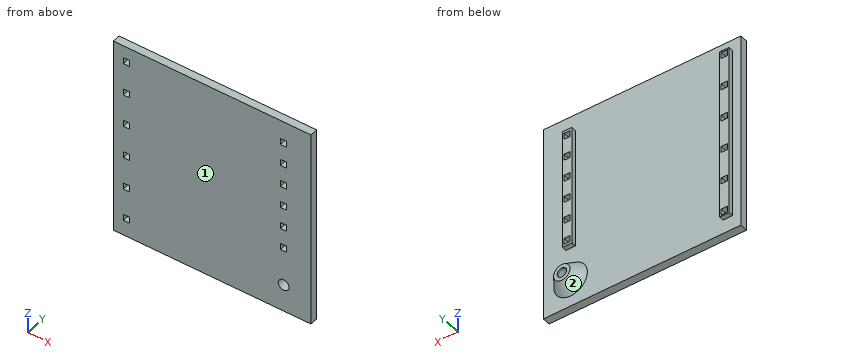
from build123d import *

# Parameters (mm, degrees)
SKETCH1_W           = 126
SKETCH1_H           = 126
BOSS_EXTRUDE1_DEPTH = 5
SKETCH3_R           = 12.5
BOSS_EXTRUDE2_DEPTH = 7.5
SKETCH4_R           = 3.45
CUT_EXTRUDE1_DEPTH  = 11.5
SKETCH6_R           = 3
CUT_EXTRUDE2_DEPTH  = 179.628805068
CHAMFER1_SIZE       = 10
CHAMFER1_SIZE_2     = 7.26542528
SKETCH9_W           = 6
SKETCH9_H           = 77
BOSS_EXTRUDE4_DEPTH = 3
SKETCH10_W          = 4
SKETCH10_H          = 4
CUT_EXTRUDE4_DEPTH  = 179.370401132
SKETCH11_W          = 6
SKETCH11_H          = 110
BOSS_EXTRUDE5_DEPTH = 3
SKETCH12_W          = 4
SKETCH12_H          = 4
CUT_EXTRUDE5_DEPTH  = 179.370401132


with BuildPart() as part:
    # Sketch1 → Boss-Extrude1 (new body)
    with BuildSketch(Plane(origin=(0, 0, 0), x_dir=(1, 0, 0), z_dir=(0, 1, 0))):
        with Locations((63, 63)):
            Rectangle(SKETCH1_W, SKETCH1_H)
    extrude(amount=BOSS_EXTRUDE1_DEPTH)

    # Sketch3 → Boss-Extrude2 (add)
    with BuildSketch(Plane(origin=(0, 5, 0), x_dir=(1, 0, 0), z_dir=(0, 1, 0))):
        with Locations(Location((108.6, 108.6, 0), (0, 0, 90))):
            Circle(SKETCH3_R)
    extrude(amount=BOSS_EXTRUDE2_DEPTH)

    # Sketch4 → Cut-Extrude1 (cut)
    with BuildSketch(Plane.XZ):
        with Locations(Location((108.6, -108.6, 0), (0, 0, 270))):
            Circle(SKETCH4_R)
    extrude(amount=-CUT_EXTRUDE1_DEPTH, mode=Mode.SUBTRACT)

    # Sketch6 → Cut-Extrude2 (cut, through all)
    with BuildSketch(Plane(origin=(0, 12.5, 0), x_dir=(1, 0, 0), z_dir=(0, 1, 0))):
        with Locations(Location((108.6, 108.6, 0), (0, 0, 270))):
            Circle(SKETCH6_R)
    extrude(amount=-CUT_EXTRUDE2_DEPTH, mode=Mode.SUBTRACT)

    # Chamfer1
    # the kernel refuses this chamfer: 10, 7.26542528 mm, written as the material it takes off along each edge
    with BuildSketch(Plane(origin=(108.6, 12.5, -108.6), x_dir=(0, 0, -1), z_dir=(1, 0, 0))) as chamfer1_piece_1_section:
        Polygon((12.5, -CHAMFER1_SIZE), (12.5 - CHAMFER1_SIZE_2, 0), (12.5, 0), align=None)
    chamfer1_piece_1 = revolve(axis=Axis((108.6, 12.5, -108.6), (0, 1, 0)), mode=Mode.PRIVATE)
    chamfer1_piece_1 = split(chamfer1_piece_1, bisect_by=Plane(origin=(108.6, 5, -100.650989912), z_dir=(0, 1, 0)), keep=Keep.TOP, mode=Mode.PRIVATE)
    add(chamfer1_piece_1, mode=Mode.SUBTRACT)

    # Sketch9 → Boss-Extrude4 (add)
    with BuildSketch(Plane(origin=(0, 5, 0), x_dir=(1, 0, 0), z_dir=(0, 1, 0))):
        with Locations((108.6, 48.95817816)):
            Rectangle(SKETCH9_W, SKETCH9_H)
    extrude(amount=BOSS_EXTRUDE4_DEPTH)

    # Sketch10 → Cut-Extrude4 (cut, through all)
    with BuildSketch(Plane(origin=(0, 8, 0), x_dir=(1, 0, 0), z_dir=(0, 1, 0))):
        with Locations((108.6, 83.95817816)):
            Rectangle(SKETCH10_W, SKETCH10_H)
        with Locations((108.6, 69.958932274)):
            Rectangle(SKETCH10_W, SKETCH10_H)
        with Locations((108.6, 55.959686388)):
            Rectangle(SKETCH10_W, SKETCH10_H)
        with Locations((108.6, 41.960440502)):
            Rectangle(SKETCH10_W, SKETCH10_H)
        with Locations((108.6, 27.961194616)):
            Rectangle(SKETCH10_W, SKETCH10_H)
        with Locations((108.6, 13.96194873)):
            Rectangle(SKETCH10_W, SKETCH10_H)
    extrude(amount=-CUT_EXTRUDE4_DEPTH, mode=Mode.SUBTRACT)

    # Sketch11 → Boss-Extrude5 (add)
    with BuildSketch(Plane(origin=(0, 5, 0), x_dir=(1, 0, 0), z_dir=(0, 1, 0))):
        with Locations((8.381061813, 62)):
            Rectangle(SKETCH11_W, SKETCH11_H)
    extrude(amount=BOSS_EXTRUDE5_DEPTH)

    # Sketch12 → Cut-Extrude5 (cut, through all)
    with BuildSketch(Plane(origin=(0, 8, 0), x_dir=(1, 0, 0), z_dir=(0, 1, 0))):
        with Locations((8.381061813, 114.236582212)):
            Rectangle(SKETCH12_W, SKETCH12_H)
        with Locations((8.381061813, 93.358892092)):
            Rectangle(SKETCH12_W, SKETCH12_H)
        with Locations((8.381061813, 72.481201972)):
            Rectangle(SKETCH12_W, SKETCH12_H)
        with Locations((8.381061813, 51.603511852)):
            Rectangle(SKETCH12_W, SKETCH12_H)
        with Locations((8.381061813, 30.725821731)):
            Rectangle(SKETCH12_W, SKETCH12_H)
        with Locations((8.381061813, 9.848131611)):
            Rectangle(SKETCH12_W, SKETCH12_H)
    extrude(amount=-CUT_EXTRUDE5_DEPTH, mode=Mode.SUBTRACT)


solid = part.part
Work out the finished part from the listing and answer in its coordinate system (mm). Face numbers are marked on the shaded views. Coordinates: 2 decimals unless noted, no trailing zeros. Loops run counter-clockwise (first coordinate to the right, second up) from the corner with the lowest first, then second, coordinate; pieces in that order, holes last. Notation, with made-up numbers: M 52,5.5 L 90,5.5 A17 ccw 90,32.5 Z; hole C 20.5,-3.5 d5. An arc over 180 degrees is marked long. Answer in a Markdown table with one row per item. Add a question column.
1. Find section C-C, the plane z = -78.5. Write down the section's boundary in (x, y).
2. Find section D-D, the plane x = 66. Write down the section's boundary in (y, z).
3. Find section A-A, the plane z = -108.6. Write down the section's boundary in (x, y).
4. Consider L1, parallel to X at y = 4, z = -108.6; L2, parallel to X at y = 6.5, z = -34; L3, parallel to Y at x = 99.5, z = -93. Determine where each line is inside the solid, lowest interval first.
5. Flat-ended cylindrical pins translate along their axes: P1, Ø1.5, axis at y = 10, z = -111.5, coming from the -X side; P2, Ø2.5, axis at x = 109.5, y = 6.5, coming from the -Z side; P3, Ø2, axis at x = 37.5, z = -71.5, coming from the +Y side. Find the tip coordinate at first contact, or state that the pin passes through.
6. The mould has two halves that part along X. Classify the marked faces 1 and 2: pulls with the +X half, pulls with the -X half, needs draft (parallel to the pull), parting line crosses it, or undercut.
7. Find section B-B, the plane x = 108.6. State how many separate pieces and enclosed holes the cut face has, then the cut area to 3 significant figures.
Reported:
| question | item | result |
|---|---|---|
| 1 | outline | M 0,0 L 126,0 L 126,5 L 111.6,5 L 111.6,8 L 105.6,8 L 105.6,5 L 11.38,5 L 11.38,8 L 5.38,8 L 5.38,5 L 0,5 Z |
| 2 | outline | M 0,-126 L 5,-126 L 5,0 L 0,0 Z |
| 3 | outline | M 0,0 L 105.15,0 L 105.15,11.5 L 105.6,11.5 L 105.6,12.5 L 103.37,12.5 L 97.92,5 L 11.38,5 L 11.38,8 L 5.38,8 L 5.38,5 L 0,5 Z; M 111.6,11.5 L 112.05,11.5 L 112.05,0 L 126,0 L 126,5 L 119.28,5 L 113.83,12.5 L 111.6,12.5 Z |
| 4 | L1 | x = 0 to 105.15, 112.05 to 126 |
| 4 | L2 | x = 5.38 to 11.38, 105.6 to 111.6 |
| 4 | L3 | y = 0 to 5 |
| 5 | P1 | stops at x = 101.51 |
| 5 | P2 | stops at z = -119.07 |
| 5 | P3 | stops at y = 5 |
| 6 | face 1 | needs draft |
| 6 | face 2 | undercut |
| 7 | separate pieces | 8 |
| 7 | enclosed holes | 0 |
| 7 | area | 703 mm^2 |
